Autodesk Inventor part; units mm, degrees
ref_plane "Work Plane3" through (0, 0, 327.1) normal (0, 0, 1) x (1, 0, 0)
ref_plane "YZ Plane" through (0, 0, 0) normal (1, 0, 0) x (0, 1, 0)
ref_plane "XZ Plane" through (0, 0, 0) normal (0, 1, 0) x (-1, 0, 0)
sketch "Sketch1" plane through (0, 0, 0) normal (0, 0, 1) x (1, 0, 0)
  circle A0 centre (0, 0) radius 228.6
  dimension "d0" = 457.2
extrude "Extrusion1" add sketch "Sketch1" along normal blind 12.7
sketch "Sketch2" plane through (0, 0, 12.7) normal (0, 0, 1) x (1, 0, 0)
  circle A0 centre (0, 0) radius 228.6
  circle A1 centre (0, 0) radius 215.9
  dimension "d3" = 457.2
  dimension "d4" = 431.8
extrude "Extrusion2" add sketch "Sketch2" along normal blind 914.4
sketch "Sketch3" plane through (0, 0, 12.7) normal (0, 0, 1) x (1, 0, 0)
  line L0 (0, -139.7) -> (164.6108, -139.7)
  line L1 (0, -127) -> (174.5961, -127)
  circle A0 centre (0, 0) radius 215.9
  circle A1 centre (0, 0) radius 215.9
  line L2 (0, 127) -> (174.5961, 127)
  line L3 (0, 139.7) -> (164.6108, 139.7)
  line L4 (0, 139.7) -> (-164.6108, 139.7)
  line L5 (0, 127) -> (-174.5961, 127)
  circle A2 centre (0, 0) radius 215.9
  line L6 (0, -127) -> (-174.5961, -127)
  line L7 (0, -139.7) -> (-164.6108, -139.7)
  dimension "d7" = 12.7
  dimension "d8" = 127
  dimension "d9" = 12.7
  dimension "d10" = 127
extrude "Extrusion3" add sketch "Sketch3" along normal blind 914.4 contours L7 A0 L6 L1 L0 | A0 L4 L3 L2 L5
ref_plane "Work Plane3" through (0, 0, 327.1) normal (0, 0, 1) x (1, 0, 0)
sketch "Sketch10" plane through (0, 0, 327.1) normal (0, 0, 1) x (1, 0, 0)
  circle A0 centre (0, 0) radius 228.6
  arc A1 (-164.6108, -139.7) -> (164.6108, -139.7) centre (0, 0) ccw
  line L0 (-164.6108, -139.7) -> (-180.9471, -139.7)
  line L1 (164.6108, -139.7) -> (-164.6108, -139.7)
  line L2 (164.6108, -139.7) -> (180.9471, -139.7)
  arc A2 (-180.9471, -139.7) -> (180.9471, -139.7) centre (0, 0) ccw
  arc A3 (164.6108, 139.7) -> (-164.6108, 139.7) centre (0, 0) ccw
  line L3 (164.6108, 139.7) -> (180.9471, 139.7)
  line L4 (-164.6108, 139.7) -> (164.6108, 139.7)
  line L5 (-164.6108, 139.7) -> (-180.9471, 139.7)
  arc A4 (180.9471, 139.7) -> (-180.9471, 139.7) centre (0, 0) ccw
  line L6 (-164.6108, 139.7) -> (164.6108, 139.7)
  line L7 (-164.6108, -139.7) -> (164.6108, -139.7)
extrude "Extrusion7" cut sketch "Sketch10" along normal through all contours L3 A3 L5 A0 | A0 L0 A1 L2 | L4 A3 | A1 L1
sketch "Sketch11" plane through (0, 0, 327.1) normal (0, 0, 1) x (1, 0, 0)
  line L0 (-180.9471, -139.7) -> (180.9471, -139.7)
  arc A0 (-180.9471, -139.7) -> (180.9471, -139.7) centre (0, 0) ccw
  arc A1 (-180.9471, -139.7) -> (180.9471, -139.7) centre (0, 0) ccw
  line L1 (-180.9471, 139.7) -> (-164.6108, 139.7)
  line L2 (-180.9471, 139.7) -> (180.9471, 139.7)
  line L3 (164.6108, 139.7) -> (180.9471, 139.7)
  arc A2 (180.9471, 139.7) -> (-180.9471, 139.7) centre (0, 0) ccw
extrude "Extrusion8" add sketch "Sketch11" against normal blind 10
properties part number "Chassis" material "ABS Plastic"
For this review, take the finished solid that the model builds, in its own axes (mm). A direction names the side the tool comes from. Coordinates: 2 decimals unless noted, no trailing zeros. Loops run counter-clockwise (first coordinate to the right, second up) from the corner with the lowest first, then second, coordinate; pieces in that order, holes last. Notation, with made-up numbers: (-31, 66) - (-24, 66) arc R17 cw to (-24, 75) - close; hole circle Ø2 at (-5.75, 20.5). An arc over 180 degrees is marked (long way). Use a Markdown table: item, result. Add a question column.
Item 1: We need section A-A (x = 0). Give the boundary of the cut face in (y, z).
Item 2: Mouldability with a two-part tool opening along X and no side actions: class faces 4 (the face through (-3, 3, 0)), 5 (the face through (-3, 2, 12.7)), 6 (the face through (2, -127, 463)) as pulls with the +X half, pulls with the -X half, needs draft (parallel to the pull), parting line crosses it, or undercut.
Item 3: We need section C-C (z = 698.5). Give the boundary of the cut face in (x, y), and give its area (3 significant figures).
Item 4: Tool access review of faces 1 (the face through (-215.89, -1.9, 463.5)), 2 (the face through (-2, -169, 12.7)), 3 (the face through (3, -139.7, 623)): name each direction out of +Z, -Z, +X, -X, +Y, -Y from which nothing blocks a thin tool from reaching the whole face with its end or side.
Item 5: We need section D-D (y = 200). Give the boundary of the cut face in (x, z), and give its area (3 significant figures).
Item 6: We need section B-B (y = 0). Give the boundary of the cut face in (x, z).
Item 7: Insertion check: pin 1 Ø1.5 at (y, z) = (-10.5, 654.5) entering from -X; pin 2 Ø10 at (x, z) = (100.5, 823.5) entering from -Y; pin 3 Ø10 at (x, z) = (108.5, 378.5) entering from +Y. Each pin has a flat end and moves straight along its axis. Give the tip position at first contact, or say it passes through.
Item 8: For line 1 (Y direction, x = -55, z = 862); line 2 (Z direction, x = 53.5, y = -191.5); line 3 (X direction, y = -0.5, z = 667), list the stretches that pass through material, from the lowest coordinate up.
Results list:
| question | item | result |
|---|---|---|
| 1 | outline | (-228.6, 0) - (228.6, 0) - (228.6, 327.1) - (139.7, 327.1) - (139.7, 927.1) - (127, 927.1) - (127, 12.7) - (-127, 12.7) - (-127, 927.1) - (-139.7, 927.1) - (-139.7, 327.1) - (-228.6, 327.1) - close; hole (-215.9, 12.7) - (-139.7, 12.7) - (-139.7, 317.1) - (-215.9, 317.1) - close; hole (139.7, 12.7) - (215.9, 12.7) - (215.9, 317.1) - (139.7, 317.1) - close |
| 2 | face 4 | needs draft |
| 2 | face 5 | undercut |
| 2 | face 6 | undercut |
| 3 | outline | (-180.95, -139.7) - (180.95, -139.7) arc R228.6 ccw to (180.95, 139.7) - (-180.95, 139.7) arc R228.6 ccw to start; hole (-174.6, -127) - (174.6, -127) arc R215.9 ccw to (174.6, 127) - (-174.6, 127) arc R215.9 ccw to start |
| 3 | area | 16,300 mm^2 |
| 4 | face 1 | +Z |
| 4 | face 2 | none |
| 4 | face 3 | +Z, +X, -X, -Y |
| 5 | outline | (-110.72, 0) - (110.72, 0) - (110.72, 327.1) - (-110.72, 327.1) - close; hole (-81.32, 12.7) - (81.32, 12.7) - (81.32, 317.1) - (-81.32, 317.1) - close |
| 5 | area | 22,900 mm^2 |
| 6 | outline | (-228.6, 0) - (228.6, 0) - (228.6, 927.1) - (215.9, 927.1) - (215.9, 12.7) - (-215.9, 12.7) - (-215.9, 927.1) - (-228.6, 927.1) - close |
| 7 | pin 1 | stops at x = -228.39 |
| 7 | pin 2 | stops at y = -139.7 |
| 7 | pin 3 | stops at y = 139.7 |
| 8 | line 1 | y = -139.7 to -127, 127 to 139.7 |
| 8 | line 2 | z = 0 to 12.7, 317.1 to 327.1 |
| 8 | line 3 | x = -228.6 to -215.9, 215.9 to 228.6 |
